Design review of the part shown in the three views and the two pictorial views. Dimensions are in mm from the part's minimum x, y and z. A direction names the side the tool comes from. Give positions to 0.01 mm unless a question says otherwise; leave off trailing zeros. Order: outer loops, then holes, each group sorted by start corner. A loop starts at its lowest first (then second) coordinate and runs counter-clockwise, first axis right, second up.
Item 1: Consider section B-B (y = 588.5). Give the boundary of the cut face in (x, z).
Item 2: Consider section A-A (z = 63.5). Give the boundary of the cut face in (x, y), plus the area to 3 significant figures.
Item 3: Machinability: for the marked faces 5, 6 and 7, which of the approach directions +Z, -Z, +X, -X, +Y, -Y give a long, thin tool a straight path to every point of the face, cutting with its end or side? Answer none if there is none.
Item 4: For P1, Ø4, axis at x = 556.5, z = 613.5, coming from the -Y side; P2, Ø25, axis at x = 497.5, y = 36, coming from the -Z side, all flat-tipped, find the tip position at first contact; note any pin that passes through.
Item 5: Consider section C-C (x = 930). Give the boundary of the cut face in (y, z).
Item 6: For probe 1 along Y at (x, z) = (735.5, 608); probe 2 along X at (y, z) = (399.5, 603); probe 3 along Z at (x, y) = (984.5, 157), list the stretches that pass through material, from the lowest coordinate up.
Item 7: The part is to be moulded in two halves that separate along Y. For the marked faces 1, 2, 3 and 4, say which applies: released by +Y, released by -Y, zero draft, split by the parting line, or undercut.
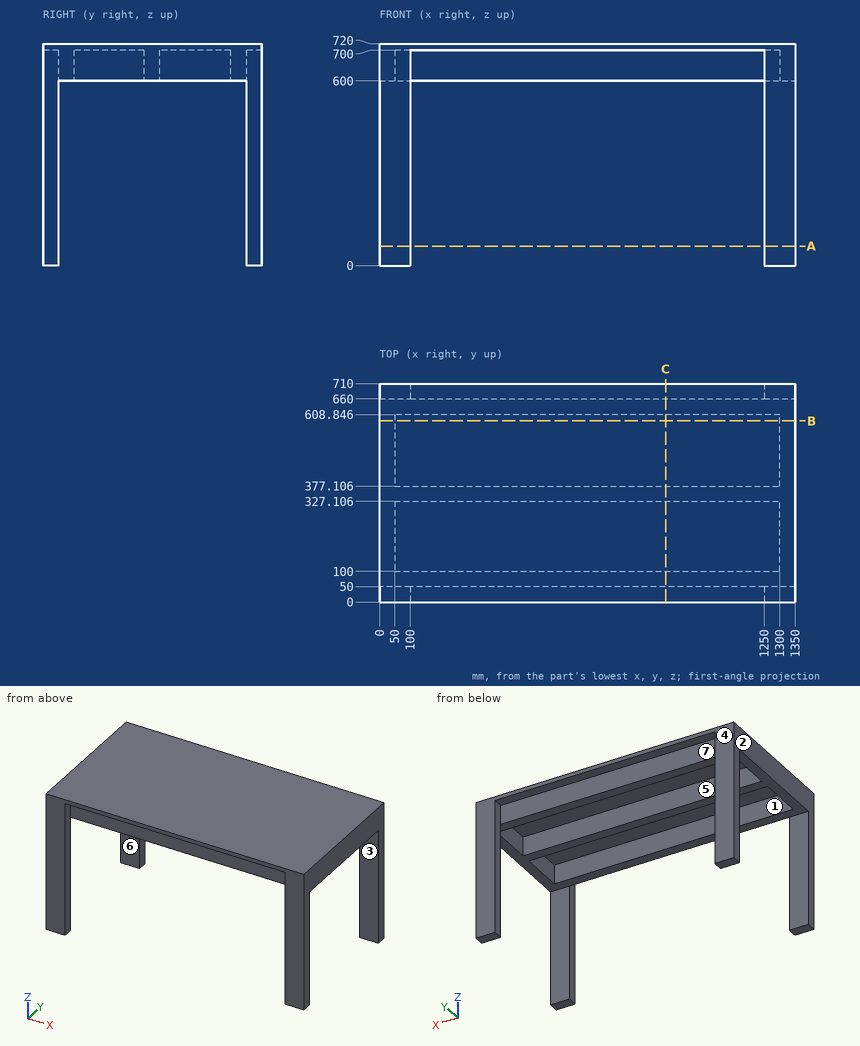
Resolved:
1. outline: (0, 600) - (50, 600) - (50, 700) - (1300, 700) - (1300, 600) - (1350, 600) - (1350, 720) - (0, 720) - close
2. outline: (0, 0) - (100, 0) - (100, 50) - (0, 50) - close; (0, 660) - (100, 660) - (100, 710) - (0, 710) - close; (1250, 0) - (1350, 0) - (1350, 50) - (1250, 50) - close; (1250, 660) - (1350, 660) - (1350, 710) - (1250, 710) - close
2. area: 20,000 mm2
3. face 5: -Z
3. face 6: -Z, +X, -X
3. face 7: -Z, +Y
4. P1: stops at y = 50
4. P2: stops at z = 700
5. outline: (0, 700) - (50, 700) - (50, 600) - (100, 600) - (100, 700) - (327.11, 700) - (327.11, 600) - (377.11, 600) - (377.11, 700) - (608.85, 700) - (608.85, 600) - (660, 600) - (660, 700) - (710, 700) - (710, 720) - (0, 720) - close
6. probe 1: y = 50 to 100, 327.11 to 377.11, 608.85 to 660
6. probe 2: x = 0 to 50, 1300 to 1350
6. probe 3: z = 700 to 720
7. face 1: undercut
7. face 2: zero draft
7. face 3: undercut
7. face 4: released by +Y
